```python
from build123d import *

# Parameters (mm, degrees)
F0_R      = 42
F0_R_2    = 36.5
F1_DEPTH  = 2
F4_R      = 42.35
F4_R_2    = 42
F5_DEPTH  = 2
F6_R      = 1.99999
F7_R      = 37.375
F7_R_2    = 34.5
F8_DEPTH  = 12
F8_TAPER  = -5
F9_R      = 38.4248639623
F10_DEPTH = 25
F11_R     = 34.5
F12_DEPTH = 25
F12_TAPER = -5
F13_R     = 1.25
F14_R     = 0.75


# Not quite as in the source:
# - a fillet or chamfer is up to 0.001 mm smaller than in the source, because OpenCascade refuses the exact size


with BuildPart() as f1:
    # F0 (on Top) → F1 (new body)
    with BuildSketch(Plane.XY):
        Circle(F0_R)
        Circle(F0_R_2, mode=Mode.SUBTRACT)
    extrude(amount=F1_DEPTH)

    # F2 (on Front) → F3 (revolve)
    with BuildSketch(Plane.XZ):
        with BuildLine():
            Line((36.5, 0), (36.5, 2))
            Line((36.5, 2), (35.5, 2))
            ThreePointArc((35.5, 2), (34.7928932188, 2.2928932188), (34.5, 3))
            Line((34.5, 3), (34.5, 14.1715728753))
            ThreePointArc((34.5, 14.1715728753), (34.6835034191, 14.7489231444), (35.1666666667, 15.1143819168))
            ThreePointArc((35.1666666667, 15.1143819168), (35.6547005384, 18.6329931619), (32.5, 17))
            Line((32.5, 17), (32.5, 2))
            ThreePointArc((32.5, 2), (33.0857864376, 0.5857864376), (34.5, 0))
            Line((34.5, 0), (36.5, 0))
        make_face()
    revolve(axis=Axis((0, 0, 63.5549128056), (0, 0, 1)))

    # F4 (on face) → F5 (join)
    with BuildSketch(Plane.XY.offset(2)):
        Circle(F4_R)
        Circle(F4_R_2, mode=Mode.SUBTRACT)
    extrude(amount=-F5_DEPTH)

    # F6 (radius 2 in the source; OpenCascade refuses exactly that, so slightly less here)
    f6_edges = [f1.edges().sort_by_distance(p)[0] for p in [
        (-42.35, 0, 2),
    ]]
    fillet(f6_edges, radius=F6_R)

    # F7 (on face) → F8 (join)
    with BuildSketch(Plane(origin=(0, 0, 0), x_dir=(1, 0, 0), z_dir=(0, 0, -1))):
        Circle(F7_R)
        Circle(F7_R_2, mode=Mode.SUBTRACT)
    extrude(amount=-F8_DEPTH, taper=F8_TAPER)

    # F9 (on face) → F10 (cut)
    with BuildSketch(Plane.XY.offset(12)):
        Circle(F9_R)
    extrude(amount=F10_DEPTH, mode=Mode.SUBTRACT)

    # F11 (on face) → F12 (cut)
    with BuildSketch(Plane(origin=(0, 0, 0), x_dir=(1, 0, 0), z_dir=(0, 0, -1))):
        Circle(F11_R)
    extrude(amount=-F12_DEPTH, taper=F12_TAPER, mode=Mode.SUBTRACT)

    # F13
    f13_edges = [f1.edges().sort_by_distance(p)[0] for p in [
        (-38.424864, 0, 12),
        (-35.549864, 0, 12),
    ]]
    fillet(f13_edges, radius=F13_R)

    # F14
    f14_edges = [f1.edges().sort_by_distance(p)[0] for p in [
        (-37.549977, 0, 2),
    ]]
    fillet(f14_edges, radius=F14_R)


solid = f1.part
```
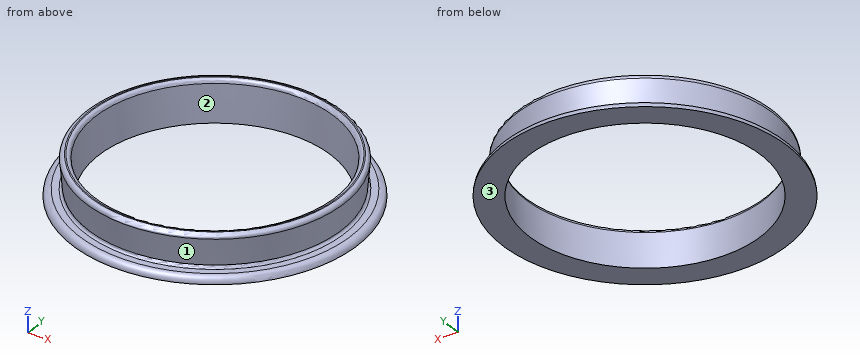
Here's how the part is built. I have some questions about the finished solid (model axes, mm). Face numbers are marked on the shaded views. Round coordinates to 2 decimals unless told otherwise and drop trailing zeros. Order: outer loops, then holes, each group sorted by start corner. A loop starts at its lowest first (then second) coordinate and runs counter-clockwise, first axis right, second up. Notation, with made-up numbers: (41.5, -39) -> (67.5, -39) arc R23 ccw to (67.5, -6) -> close; hole circle Ø2 at (57, -38). An arc over 180 degrees is marked (long way). Use a Markdown table: item, result. Add a question column.
(1) If we mould it in two halves opening along X, with no side actions, what happens to the marked faces 1, 2 and 3? For each: released by +X, released by -X, zero draft, split by the parting line, or undercut.
(2) Suppose I cut it at B-B, the plane z = 6.25. Please give me the cut outline in (x, y).
(3) I need wall thicknesses on line 1 along X through (y, z) = (-7.5, 6.5); line 2 along Y through (x, z) = (16.5, 8); line 3 along X through (y, z) = (-19, 8). Which ranges of each line are inside material? Lowest first, please.
(4) For pin 1 Ø4 at (y, z) = (-17, 8.5) entering from -X; pin 2 Ø24 at (x, y) = (15.5, -16) entering from +Z; pin 3 Ø2 at (y, z) = (-24, 4.5) entering from +X; pin 4 Ø2 at (y, z) = (-28, 2) entering from +X, each with a flat end and sliding along its axis, tell me the tip position at first contact or that it passes through.
Verdict:
| question | item | result |
|---|---|---|
| 1 | face 1 | split by the parting line |
| 1 | face 2 | undercut |
| 1 | face 3 | zero draft |
| 2 | outline | circle Ø75.84 at (0, 0); hole circle Ø70.09 at (0, 0) |
| 3 | line 1 | -37.2 to -34.26, 34.26 to 37.2 |
| 3 | line 2 | -34.31 to -31.09, 31.09 to 34.31 |
| 3 | line 3 | -33 to -29.63, 29.63 to 33 |
| 4 | pin 1 | x = -35.06 |
| 4 | pin 2 | through |
| 4 | pin 3 | x = 29.97 |
| 4 | pin 4 | x = 31.77 |
